Read the model definition and answer for the solid it produces. Units are mm, in the model's axes. Face numbers are marked on the shaded views. A direction names the side the tool comes from. Give positions to 0.01 mm unless a question says otherwise; leave off trailing zeros. Write each loop counter-clockwise with the first axis right and the second up, starting at its lowest first coordinate (ties: lowest second). Pieces come first, ordered by that corner, then holes.
```python
from build123d import *

# Parameters (mm, degrees)
SKETCH2_W          = 1
SKETCH2_H          = 6.5
CUT_EXTRUDE1_DEPTH = 1.5


with BuildPart() as part:
    # Sketch1 → Revolve1 (revolve)
    with BuildSketch(Plane.XY):
        Polygon((0, 0), (-33, 0), (-33, 2), (-3, 2), (-3, 3.25), (0, 3.25), align=None)
    revolve(axis=Axis((0, 0, 0), (-1, 0, 0)))

    # Sketch2 → Cut-Extrude1 (cut)
    with BuildSketch(Plane(origin=(0, 0, 0), x_dir=(0, 0, -1), z_dir=(1, 0, 0))):
        Rectangle(SKETCH2_W, SKETCH2_H)
    extrude(amount=-CUT_EXTRUDE1_DEPTH, mode=Mode.SUBTRACT)


solid = part.part
```
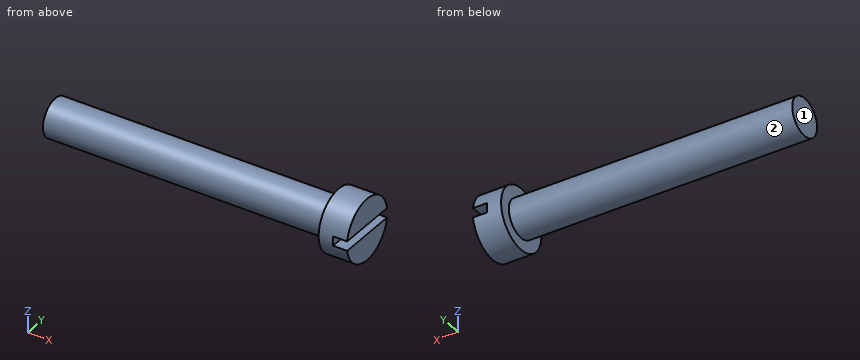
Item 1: Find the intervals of material crossed by line 1 along X through (y, z) = (-0.25, 3); line 2 along Y through (x, z) = (-6.5, 0); line 3 along Z through (x, y) = (-1, -1.5), in increasing order.
Result set:
line 1: x = -3 to 0
line 2: y = -2 to 2
line 3: z = -2.88 to -0.5, 0.5 to 2.88
Item 2: Section A-A (y = 0) is taken. Write down the section's boundary in (x, z).
Result set:
outline: (-33, -2) - (-3, -2) - (-3, -3.25) - (0, -3.25) - (0, -0.5) - (-1.5, -0.5) - (-1.5, 0.5) - (0, 0.5) - (0, 3.25) - (-3, 3.25) - (-3, 2) - (-33, 2) - close
Item 3: Section D-D (y = -1.5) is taken. Write down the section's boundary in (x, z), and give its area (3 significant figures).
Result set:
outline: (-33, -1.32) - (-3, -1.32) - (-3, -2.88) - (0, -2.88) - (0, -0.5) - (-1.5, -0.5) - (-1.5, 0.5) - (0, 0.5) - (0, 2.88) - (-3, 2.88) - (-3, 1.32) - (-33, 1.32) - close
area: 95.2 mm2
Item 4: Section B-B (z = 0) is taken. Write down the section's boundary in (x, y).
Result set:
outline: (-33, -2) - (-3, -2) - (-3, -3.25) - (-1.5, -3.25) - (-1.5, 3.25) - (-3, 3.25) - (-3, 2) - (-33, 2) - close
Item 5: Which of the six approach directions +Z, -Z, +X, -X, +Y, -Y give full straight-line access (tool end or side, diameter ignored) to the marked faces 1 and 2?
Result set:
face 1: +Z, -Z, -X, +Y, -Y
face 2: -X
Item 6: Section C-C (x = -2.5) is taken. Write down the section's boundary in (y, z), and give its area (3 significant figures).
Result set:
outline: circle Ø6.5 at (0, 0)
area: 33.2 mm2
Item 7: Each of these flat-tipped pins is pushed along its axis until it touches: pin 1 Ø1.2 at (x, y) = (-0.5, -1) entering from -Z; pin 2 Ø2 at (x, z) = (-21.5, 2.5) entering from +Y; pin 3 Ø0.8 at (y, z) = (1, 0) entering from +X. Where does it stop, or does it pass through?
Result set:
pin 1: stops at z = -3.23
pin 2: stops at y = 1.32
pin 3: stops at x = -1.5
